The model under review builds one solid part; all positions refer to its coordinate system, in mm. Face numbers are marked on the shaded views. A direction names the side the tool comes from. Coordinates: 2 decimals unless noted, no trailing zeros. Loops run counter-clockwise (first coordinate to the right, second up) from the corner with the lowest first, then second, coordinate; pieces in that order, holes last. Notation, with made-up numbers: M 78,41.5 L 110,41.5 A16 cw 110,58.5 Z; hole C 58.5,4 d10. An arc over 180 degrees is marked long. One line per item, written item: value.
```python
from build123d import *

# Parameters (mm, degrees)
EXTRUDE_1_DEPTH     = 8.5
SKETCH_3_R          = 3.25
CUT_EXTRUDE_1_DEPTH = 54.826108906
SKETCH_4_R          = 3.25
CUT_EXTRUDE_2_DEPTH = 54.826108906


with BuildPart() as part:
    # 草图1 → 凸台-拉伸1 (new, symmetric)
    with BuildSketch(Plane.XY):
        Polygon((0, 0), (40, 0), (40, 40), (37.5, 40), (35, 30), (35, 24.364950833), (35.6, 23.764950833), (35, 23.164950833), (35, 21.364950833), (35.6, 20.764950833), (35, 20.164950833), (35, 13), (27, 5), (19.835049167, 5), (19.235049167, 4.4), (18.635049167, 5), (16.835049167, 5), (16.235049167, 4.4), (15.635049167, 5), (10, 5), (0, 2.5), align=None)
    extrude(amount=EXTRUDE_1_DEPTH, both=True)

    # 草图3 → 切除-拉伸1 (cut, through all)
    with BuildSketch(Plane(origin=(0, 5, 0), x_dir=(1, 0, 0), z_dir=(0, 1, 0))):
        with Locations(Location((20, 0, 0), (0, 0, 270))):
            Circle(SKETCH_3_R)
    extrude(amount=-CUT_EXTRUDE_1_DEPTH, mode=Mode.SUBTRACT)

    # 草图4 → 切除-拉伸2 (cut, through all)
    with BuildSketch(Plane.ZY.offset(-35)):
        with Locations((0, 20)):
            Circle(SKETCH_4_R)
    extrude(amount=-CUT_EXTRUDE_2_DEPTH, mode=Mode.SUBTRACT)


solid = part.part
```
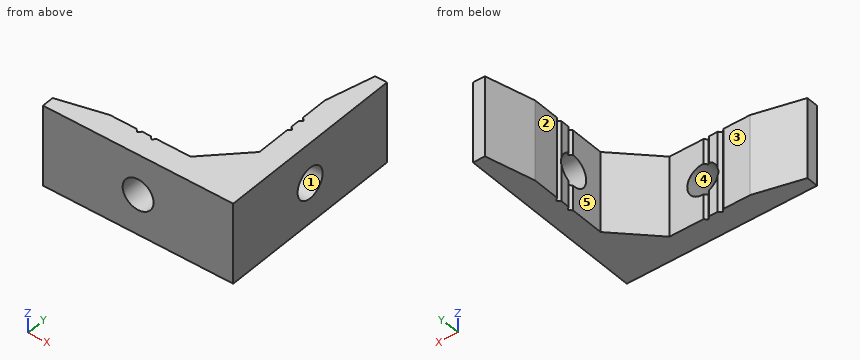
(1) Insertion check: pin 1 Ø1.7 at (y, z) = (27, 2) entering from -X; pin 2 Ø1.5 at (y, z) = (13, -2.5) entering from -X; pin 3 Ø2 at (x, z) = (23.5, -2.5) entering from +Y; pin 4 Ø2 at (x, z) = (4.5, -3.5) entering from -Y. Each pin has a flat end and moves straight along its axis. Give the tip position at first contact, or say it passes through.
Checks:
pin 1: x = 35
pin 2: x = 34.25
pin 3: y = 5
pin 4: y = 0
(2) Add section C-C on y = 10.5. State the section outline as (x, z) points, then the cut area to 4 significant figures.
Checks:
outline: M 32.5,-8.5 L 40,-8.5 L 40,8.5 L 32.5,8.5 Z
area: 127.5 mm^2
(3) To check wall thickness, follow L1, parallel to Z at x = 20, y = 3.2; L2, parallel to X at y = 1.2, z = 0; L3, parallel to X at y = 30, z = -3. State the ranges of each line that lie inside material, in increasing order. Write a range as [from, to].
Checks:
L1: [-8.5, -3.25], [3.25, 8.5]
L2: [0, 16.75], [23.25, 40]
L3: [35, 40]
(4) Tool access review of the marked faces 1 and 2: name each direction out of +Z, -Z, +X, -X, +Y, -Y from which nothing blocks a thin tool from reaching the whole face with its end or side.
Checks:
face 1: +X, -X
face 2: +Z, -Z, -X, +Y
(5) Draft analysis for pull direction X (two halves, no side actions). For the marked faces 3, 4 and 5, state which applies: pulls with the +X half, pulls with the -X half, needs draft (parallel to the pull), parting line crosses it, or undercut.
Checks:
face 3: needs draft
face 4: undercut
face 5: pulls with the -X half
(6) Add section B-B on x = 32.5. State the section outline as (y, z) points.
Checks:
outline: M 0,-8.5 L 10.5,-8.5 L 10.5,8.5 L 0,8.5 Z
(7) Add section A-A on z = 1.25. State the section outline as (x, y) points.
Checks:
outline: M 0,0 L 17,0 L 17,5 L 16.84,5 L 16.24,4.4 L 15.64,5 L 10,5 L 0,2.5 Z; M 23,0 L 40,0 L 40,17 L 35,17 L 35,13 L 27,5 L 23,5 Z; M 35,23 L 40,23 L 40,40 L 37.5,40 L 35,30 L 35,24.36 L 35.6,23.76 L 35,23.16 Z
